from build123d import *

# Parameters (mm, degrees)
F1_W      = 367
F1_H      = 367
F2_DEPTH  = 100
F3_W      = 347
F3_H      = 347
F4_DEPTH  = 100.001
F6_W      = 357
F6_H      = 362
F7_DEPTH  = 3.5
F9_W      = 357
F9_H      = 357
F10_DEPTH = 3
F12_W     = 357
F12_H     = 362
F13_DEPTH = 3.5


with BuildPart() as f2:
    # F1 (on Front) → F2 (new body)
    with BuildSketch(Plane.XZ):
        Rectangle(F1_W, F1_H)
    extrude(amount=-F2_DEPTH)

    # F3 (on Front) → F4 (cut, through all)
    with BuildSketch(Plane.XZ):
        Rectangle(F3_W, F3_H)
    extrude(amount=-F4_DEPTH, mode=Mode.SUBTRACT)

    # F6 (on offset) → F7 (cut)
    with BuildSketch(Plane.XZ.offset(-5)):
        with Locations((0, 2.5)):
            Rectangle(F6_W, F6_H)
    extrude(amount=-F7_DEPTH, mode=Mode.SUBTRACT)

    # F9 (on offset) → F10 (cut)
    with BuildSketch(Plane.XZ.offset(-95)):
        Rectangle(F9_W, F9_H)
    extrude(amount=F10_DEPTH, mode=Mode.SUBTRACT)

    # F12 (on offset) → F13 (cut)
    with BuildSketch(Plane.XZ.offset(-16.5)):
        with Locations((0, 2.5)):
            Rectangle(F12_W, F12_H)
    extrude(amount=-F13_DEPTH, mode=Mode.SUBTRACT)


solid = f2.part
Work out the finished part from the listing and answer in its coordinate system (mm). A direction names the side the tool comes from. Round coordinates to 2 decimals unless told otherwise and drop trailing zeros. Loops run counter-clockwise (first coordinate to the right, second up) from the corner with the lowest first, then second, coordinate; pieces in that order, holes last. Notation, with made-up numbers: (-7, -35) - (26, -35) arc R26 ccw to (26, -19) - close; hole circle Ø2 at (-4, -19.75). An arc over 180 degrees is marked (long way). Use one line per item in the form item = value. Start each with the question number.
(1) Determine the mould class of faces 4 (the face through (-2, 55, -173.5)), 5 (the face through (183.5, 49, -3)), 6 (the face through (-2, 12, -173.5)), 7 (the face through (-3, 49, 183.5)) for opening direction X: +X half, -X half, draft (parallel to the pull), parting line (faces both ways), or undercut.
(2) Which of the six approach directions +Z, -Z, +X, -X, +Y, -Y give full straight-line access (tool end or side, diameter ignored) to faces 1 (the face through (-183.5, 49, -3)), 2 (the face through (-1, 5, 178)), 3 (the face through (-173.5, 55, -2))?
(3) A flat-ended cylindrical pin translates along its axis: P1, Ø1.8, axis at x = -75.5, y = 6.5, coming from the +Z side. Find the tip coordinate at first contact, or state that the pin passes through.
(4) Consider line 1 (X direction, y = 41, z = -123); line 2 (Z direction, x = -59.5, y = 92.5). Determine where each line is inside the solid, lowest interval first.
(5) Find section C-C on y = 70.5. Determine the outline of the cut face in (x, z).
(6) Find section A-A on x = -108.5. Give the number of separate pieces and of enclosed holes in the cut face, and give its area (4 significant figures).
Answer list:
q1.face_4 = undercut
q1.face_5 = +X half
q1.face_6 = undercut
q1.face_7 = draft
q2.face_1 = +Z, -Z, -X, +Y, -Y
q2.face_2 = +Z
q2.face_3 = +Y, -Y
q3.P1 = -178.5
q4.line_1 = -183.5 to -173.5, 173.5 to 183.5
q4.line_2 = -183.5 to -178.5, 178.5 to 183.5
q5.outline = (-183.5, -183.5) - (183.5, -183.5) - (183.5, 183.5) - (-183.5, 183.5) - close; hole (-173.5, -173.5) - (173.5, -173.5) - (173.5, 173.5) - (-173.5, 173.5) - close
q6.separate_pieces = 4
q6.enclosed_holes = 0
q6.area = 1,865 mm^2
